```python
from build123d import *

# Parameters (mm, degrees)
FILLET1_R          = 0.5
SKETCH2_R          = 1.5
CUT_EXTRUDE1_DEPTH = 16.835087755


with BuildPart() as part:
    # Sketch1 → Revolve1 (revolve)
    with BuildSketch(Plane.XY, mode=Mode.PRIVATE) as revolve1_sk:
        Polygon((3, 0), (3, 3.4), (1.5, 3.4), (1.5, 5.5), (10.5, 5.5), (10.5, 3.5), (4.5, 3.5), (4.5, 0), align=None)
    revolve(revolve1_sk.sketch.rotate(Axis((0, 0, 0), (0, 1, 0)), 90), axis=Axis((0, 0, 0), (0, 1, 0)))

    # Fillet1
    fillet1_edges = [part.edges().sort_by_distance(p)[0] for p in [
        (0, 5.5, 10.5),
        (0, 3.5, 10.5),
        (0, 3.5, 4.5),
    ]]
    fillet(fillet1_edges, radius=FILLET1_R)

    # Sketch2 → Cut-Extrude1 (cut, through all)
    with BuildSketch(Plane(origin=(0, 5.5, 0), x_dir=(1, 0, 0), z_dir=(0, 1, 0))):
        with Locations(Location((0, 7.5, 0), (0, 0, 270))):
            Circle(SKETCH2_R)
        with Locations(Location((-7.5, 0, 0), (0, 0, 270))):
            Circle(SKETCH2_R)
        with Locations(Location((0, -7.5, 0), (0, 0, 270))):
            Circle(SKETCH2_R)
        with Locations(Location((7.5, 0, 0), (0, 0, 270))):
            Circle(SKETCH2_R)
    extrude(amount=-CUT_EXTRUDE1_DEPTH, mode=Mode.SUBTRACT)


solid = part.part
```
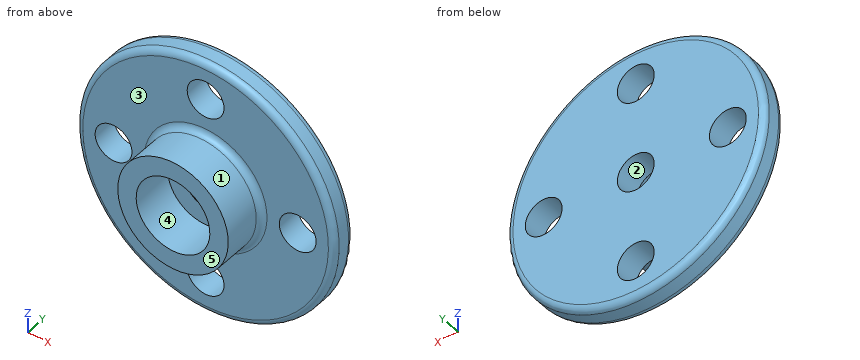
Source: CAD feature listing. Evaluate the final solid. Frame: model axes, mm. Face numbers are marked on the shaded views. A direction names the side the tool comes from. Round coordinates to 2 decimals unless told otherwise and drop trailing zeros. Loops run counter-clockwise (first coordinate to the right, second up) from the corner with the lowest first, then second, coordinate; pieces in that order, holes last. Notation, with made-up numbers: M 32.25,74.25 L 67.25,74.25 A35 ccw 67.25,110.25 Z; hole C 70,74.5 d7. An arc over 180 degrees is marked long. Use a Markdown table: item, result. Add a question column.
1. Section query A-A on x = 0. Give the number of separate pieces and of enclosed holes in the cut face, then the cut area to 3 significant figures.
2. Reachability of the marked faces 4 and 5 from +Z, -Z, +X, -X, +Y, -Y: full face, straight path, thin tool, end or side. Return the list, or none.
3. Mould query, pull axis Z, two halves, no side actions, for the marked faces 1, 2 and 3. Classes: pulls with the +Z half, pulls with the -Z half, needs draft (parallel to the pull), parting line crosses it, or undercut.
4. Section query C-C on y = 4.3. Return the cut outline in (x, z), then the cut area to 3 significant figures.
5. Line query: line 1 (X direction, y = 4.45, z = 0); line 2 (Z direction, x = -0.75, y = 4.55); line 3 (Y direction, x = 5, z = 3.25). Output: solid intervals per line, ascending.
6. Section query D-D on y = 1.65. Return the cut outline in (x, z).
7. Contact query for flat-ended pins moving along their axis: P1, Ø5, axis at x = 0, z = -7.5, coming from the -Y side; P2, Ø10, axis at x = -3.5, z = 4, coming from the -Y side; P3, Ø1.8, axis at x = 7.5, z = 0, coming from the +Y side. Output: stop coordinate, or through.
Reported:
| question | item | result |
|---|---|---|
| 1 | separate pieces | 4 |
| 1 | enclosed holes | 0 |
| 1 | area | 34.7 mm² |
| 2 | face 4 | -Y |
| 2 | face 5 | +Z, -Z, +X, -X, -Y |
| 3 | face 1 | parting line crosses it |
| 3 | face 2 | undercut |
| 3 | face 3 | needs draft |
| 4 | outline | C 0,0 d21; hole C -7.5,0 d3; hole C 0,-7.5 d3; hole C 0,0 d3; hole C 0,7.5 d3; hole C 7.5,0 d3 |
| 4 | area | 311 mm² |
| 5 | line 1 | x = -10.5 to -9, -6 to -1.5, 1.5 to 6, 9 to 10.5 |
| 5 | line 2 | z = -10.47 to -8.8, -6.2 to -1.3, 1.3 to 6.2, 8.8 to 10.47 |
| 5 | line 3 | y = 3.5 to 5.5 |
| 6 | outline | C 0,0 d9; hole C 0,0 d6 |
| 7 | P1 | stops at y = 3.5 |
| 7 | P2 | stops at y = 0 |
| 7 | P3 | passes through |
